Geometry: see drawing. Coordinates: mm, zero at the bounding-box minimum. Coordinates: 2 decimals unless noted, no trailing zeros. Loops run counter-clockwise (first coordinate to the right, second up) from the corner with the lowest first, then second, coordinate; pieces in that order, holes last.
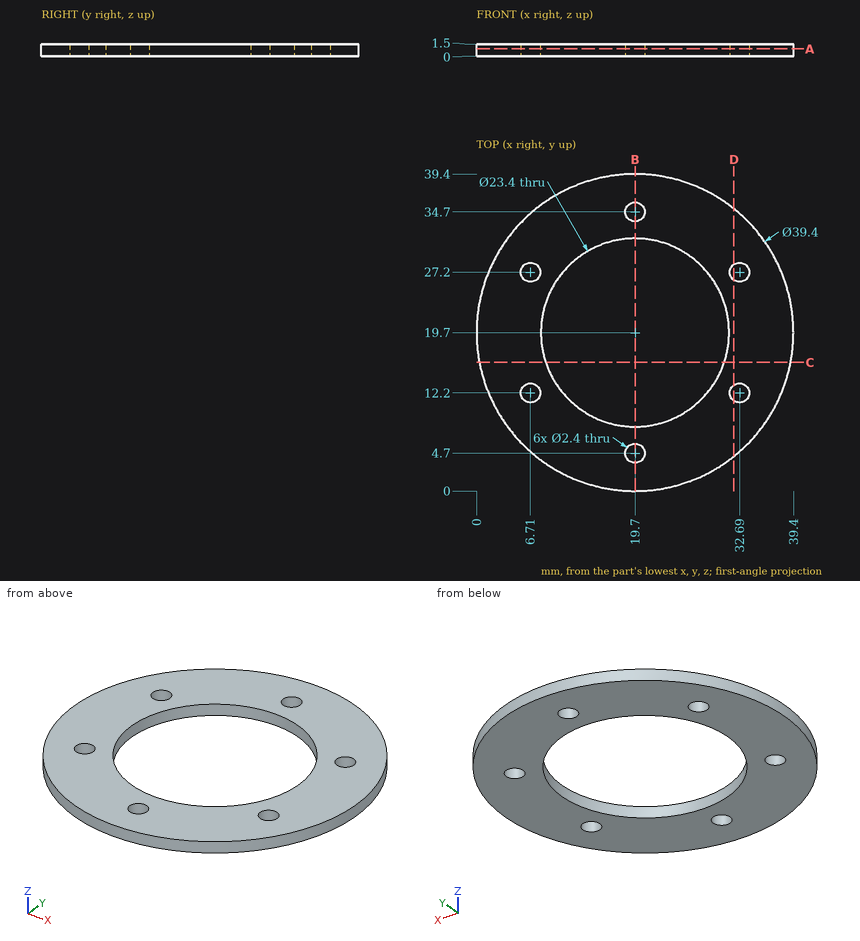
Item 1: Section query A-A (z = 0.9). Output: boundary loops of the cut face in (x, y).
Result:
outline: circle Ø39.4 at (19.7, 19.7); hole circle Ø2.4 at (6.71, 12.2); hole circle Ø2.4 at (6.71, 27.2); hole circle Ø23.4 at (19.7, 19.7); hole circle Ø2.4 at (19.7, 4.7); hole circle Ø2.4 at (19.7, 34.7); hole circle Ø2.4 at (32.69, 12.2); hole circle Ø2.4 at (32.69, 27.2)
Item 2: Contact query for a flat-ended pin moving along its axis: P1, Ø3, axis at x = 19.7, y = 34.7, coming from the +Z side. Output: stop coordinate, or through.
Result:
P1: stops at z = 1.5
Item 3: Line query: L1, parallel to Y at x = 19.7, z = 1.1; L2, parallel to X at y = 12.5, z = 0.2; L3, parallel to Y at x = 33, z = 0.2. Output: solid intervals per line, ascending.
Result:
L1: y = 0 to 3.5, 5.9 to 8, 31.4 to 33.5, 35.9 to 39.4
L2: x = 1.36 to 5.55, 7.87 to 10.48, 28.92 to 31.53, 33.85 to 38.04
L3: y = 5.17 to 11.04, 13.36 to 26.04, 28.36 to 34.23
Item 4: Section query B-B (x = 19.7). Output: boundary loops of the cut face in (y, z), then the cut area to 3 significant figures.
Result:
outline: (0, 0) - (3.5, 0) - (3.5, 1.5) - (0, 1.5) - close; (5.9, 0) - (8, 0) - (8, 1.5) - (5.9, 1.5) - close; (31.4, 0) - (33.5, 0) - (33.5, 1.5) - (31.4, 1.5) - close; (35.9, 0) - (39.4, 0) - (39.4, 1.5) - (35.9, 1.5) - close
area: 16.8 mm2
Item 5: Section query D-D (x = 32). Output: boundary loops of the cut face in (y, z).
Result:
outline: (4.31, 0) - (11.22, 0) - (11.22, 1.5) - (4.31, 1.5) - close; (13.18, 0) - (26.22, 0) - (26.22, 1.5) - (13.18, 1.5) - close; (28.18, 0) - (35.09, 0) - (35.09, 1.5) - (28.18, 1.5) - close
Item 6: Section query C-C (y = 16). Output: boundary loops of the cut face in (x, z).
Result:
outline: (0.35, 0) - (8.6, 0) - (8.6, 1.5) - (0.35, 1.5) - close; (30.8, 0) - (39.05, 0) - (39.05, 1.5) - (30.8, 1.5) - close
